For this review, take the finished solid that the model builds, in its own axes (mm). Coordinates: 2 decimals unless noted, no trailing zeros. Order: outer loops, then holes, each group sorted by start corner. A loop starts at its lowest first (then second) coordinate and runs counter-clockwise, first axis right, second up. Notation, with made-up numbers: (-10, 2.5) -> (42, 2.5) arc R24 ccw to (42, 26.5) -> close; hole circle Ø2 at (15.5, -33.75). An arc over 180 degrees is marked (long way). Return JSON: item names as keys, results as strings. Group by question number.
Item 1: Take a section at B-B (x = 27.5). Write out the cut boundary in (y, z), then the cut area to 3 significant figures.
Item 2: Take a section at C-C (y = 0.5). Write out the cut boundary in (x, z), then the cut area to 3 significant figures.
Item 3: For line 1 along X through (y, z) = (0.25, 0); line 2 along Z through (x, y) = (-1.5, 0.3); line 3 along X through (y, z) = (0.8, -27.5), list the stretches that pass through material, from the lowest coordinate up.
Item 4: Take a section at D-D (z = -27.5). Write out the cut boundary in (x, y).
Item 5: Take a section at A-A (z = 0). Write out the cut boundary in (x, y).
Item 6: Draft analysis for pull direction Z (two halves, no side actions). For faces 1 (the cylindrical face through (25.304, 0.507, -0.488)), 2 (the cylindrical face through (-21.3, 0.49, -27.77)), 3 (the flat face through (0, 0, 0)), state which applies: +Z half, -Z half, draft (parallel to the pull), parting line (faces both ways), or undercut.
```python
from build123d import *

# Parameters (mm, degrees)
SKETCH1_R           = 35
SKETCH1_R_2         = 20
BOSS_EXTRUDE1_DEPTH = 1
SKETCH3_R           = 20
BOSS_EXTRUDE2_DEPTH = 1
CUT_EXTRUDE1_REACH  = 51.508
SKETCH4_R           = 2.25


with BuildPart() as part:
    # Sketch1 → Boss-Extrude1 (new body)
    with BuildSketch(Plane(origin=(0, 0, 0), x_dir=(1, 0, 0), z_dir=(0, 1, 0))):
        with Locations(Location((0, 0, 0), (0, 0, 270))):
            Circle(SKETCH1_R)
        with Locations(Location((0, 0, 0), (0, 0, 270))):
            Circle(SKETCH1_R_2, mode=Mode.SUBTRACT)
    extrude(amount=BOSS_EXTRUDE1_DEPTH)

    # Sketch3 → Boss-Extrude2 (add)
    with BuildSketch(Plane(origin=(0, 0, 0), x_dir=(1, 0, 0), z_dir=(0, 1, 0))):
        Circle(SKETCH3_R)
    extrude(amount=BOSS_EXTRUDE2_DEPTH)

    # Sketch4 → Cut-Extrude1 (cut, up to next)
    with BuildSketch(Plane(origin=(0, 1, 0), x_dir=(1, 0, 0), z_dir=(0, 1, 0)), mode=Mode.PRIVATE) as cut_extrude1_sk1:
        with Locations(Location((0, 27.5, 0), (0, 0, 270))):
            Circle(SKETCH4_R)
    cut_extrude1_tool1 = extrude(cut_extrude1_sk1.sketch, amount=-CUT_EXTRUDE1_REACH, mode=Mode.PRIVATE) & part.part
    # Sketch4 → Cut-Extrude1 (cut, up to next)
    with BuildSketch(Plane(origin=(0, 1, 0), x_dir=(1, 0, 0), z_dir=(0, 1, 0)), mode=Mode.PRIVATE) as cut_extrude1_sk2:
        with Locations(Location((27.5, 0, 0), (0, 0, 270))):
            Circle(SKETCH4_R)
    cut_extrude1_tool2 = extrude(cut_extrude1_sk2.sketch, amount=-CUT_EXTRUDE1_REACH, mode=Mode.PRIVATE) & part.part
    # Sketch4 → Cut-Extrude1 (cut, up to next)
    with BuildSketch(Plane(origin=(0, 1, 0), x_dir=(1, 0, 0), z_dir=(0, 1, 0)), mode=Mode.PRIVATE) as cut_extrude1_sk3:
        with Locations(Location((0, -27.5, 0), (0, 0, 270))):
            Circle(SKETCH4_R)
    cut_extrude1_tool3 = extrude(cut_extrude1_sk3.sketch, amount=-CUT_EXTRUDE1_REACH, mode=Mode.PRIVATE) & part.part
    # Sketch4 → Cut-Extrude1 (cut, up to next)
    with BuildSketch(Plane(origin=(0, 1, 0), x_dir=(1, 0, 0), z_dir=(0, 1, 0)), mode=Mode.PRIVATE) as cut_extrude1_sk4:
        with Locations(Location((-27.5, 0, 0), (0, 0, 270))):
            Circle(SKETCH4_R)
    cut_extrude1_tool4 = extrude(cut_extrude1_sk4.sketch, amount=-CUT_EXTRUDE1_REACH, mode=Mode.PRIVATE) & part.part
    add(cut_extrude1_tool1.solids().sort_by_distance((0, 1, -27.5))[0], mode=Mode.SUBTRACT)
    add(cut_extrude1_tool2.solids().sort_by_distance((27.5, 1, 0))[0], mode=Mode.SUBTRACT)
    add(cut_extrude1_tool3.solids().sort_by_distance((0, 1, 27.5))[0], mode=Mode.SUBTRACT)
    add(cut_extrude1_tool4.solids().sort_by_distance((-27.5, 1, 0))[0], mode=Mode.SUBTRACT)


solid = part.part
```
Findings below:
{
 "1": {"outline": "(0, -21.65) -> (1, -21.65) -> (1, -2.25) -> (0, -2.25) -> close; (0, 2.25) -> (1, 2.25) -> (1, 21.65) -> (0, 21.65) -> close", "area": "38.8 mm2"},
 "2": {"outline": "circle Ø70 at (0, 0); hole circle Ø4.5 at (-27.5, 0); hole circle Ø4.5 at (0, -27.5); hole circle Ø4.5 at (0, 27.5); hole circle Ø4.5 at (27.5, 0)", "area": "3,780 mm2"},
 "3": {"line 1": "x = -35 to -29.75, -25.25 to 25.25, 29.75 to 35", "line 2": "z = -34.97 to -29.18, -25.82 to 25.82, 29.18 to 34.97", "line 3": "x = -21.65 to -2.25, 2.25 to 21.65"},
 "4": {"outline": "(-21.65, 0) -> (-2.25, 0) -> (-2.25, 1) -> (-21.65, 1) -> close; (2.25, 0) -> (21.65, 0) -> (21.65, 1) -> (2.25, 1) -> close"},
 "5": {"outline": "(-35, 0) -> (-29.75, 0) -> (-29.75, 1) -> (-35, 1) -> close; (-25.25, 0) -> (25.25, 0) -> (25.25, 1) -> (-25.25, 1) -> close; (29.75, 0) -> (35, 0) -> (35, 1) -> (29.75, 1) -> close"},
 "6": {"face 1": "undercut", "face 2": "parting line", "face 3": "draft"}
}
